Could you check a few things on this drawing? It's one solid part, dimensions in mm from its lowest x, y, z. A direction names the side the tool comes from. Give positions to 0.01 mm unless a question says otherwise; leave off trailing zeros. Loops run counter-clockwise (first coordinate to the right, second up) from the corner with the lowest first, then second, coordinate; pieces in that order, holes last.
Q1. Suppose I cut it at C-C (z = 7.5). List the corners of the cut face in (x, y) for me, and give its area (3 significant figures).
Q2. I need wall thicknesses on probe 1 along Z at (x, y) = (14, 30.5); probe 2 along Y at (x, z) = (14, 30) (1 decimal); probe 3 along Z at (x, y) = (36.5, 20). Which ranges of each line are inside material? Lowest first, please.
Q3. Suppose I cut it at D-D (x = 37). List the corners of the cut face in (y, z) for me.
Q4. I'm going to push flat-ended pins straight in: P1, Ø0.8, axis at x = 14.5, y = 5.5, coming from the +Z side; P2, Ø8, axis at x = 37, y = 13, coming from the +Z side; P3, Ø1.5, axis at x = 7.5, z = 22, coming from the +Y side. Where does each tip first touch, or does it pass through?
Q5. Suppose I cut it at A-A (x = 22). List the corners of the cut face in (y, z) for me, and give its area (3 significant figures).
Q6. Suppose I cut it at B-B (y = 19). List the corners of the cut face in (x, z) for me, and give its area (3 significant figures).
Q7. For the marked faces 1, 2 and 3, which set-ups out of +Z, -Z, +X, -X, +Y, -Y let a thin tool reach every point of the face, with its end or its side?
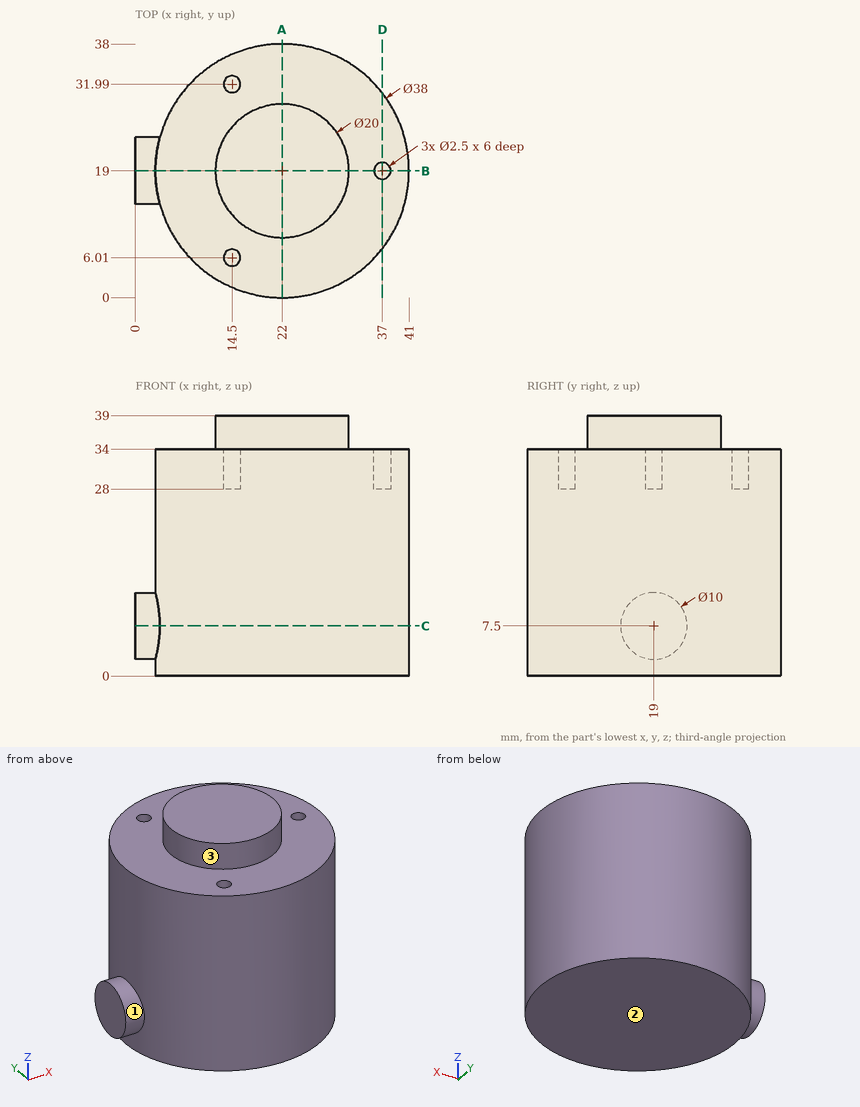
Solutions:
1. outline: (0, 14) - (3.67, 14) arc R19 ccw (long way) to (3.67, 24) - (0, 24) - close
1. area: 1,170 mm2
2. probe 1: z = 0 to 34
2. probe 2: y = 1.8 to 4.9, 7.2 to 30.8, 33.1 to 36.2
2. probe 3: z = 0 to 28
3. outline: (7.34, 0) - (30.66, 0) - (30.66, 34) - (20.25, 34) - (20.25, 28) - (17.75, 28) - (17.75, 34) - (7.34, 34) - close
4. P1: stops at z = 28
4. P2: stops at z = 34
4. P3: stops at y = 32.11
5. outline: (0, 0) - (38, 0) - (38, 34) - (29, 34) - (29, 39) - (9, 39) - (9, 34) - (0, 34) - close
5. area: 1,390 mm2
6. outline: (0, 2.5) - (3, 2.5) - (3, 0) - (41, 0) - (41, 34) - (38.25, 34) - (38.25, 28) - (35.75, 28) - (35.75, 34) - (32, 34) - (32, 39) - (12, 39) - (12, 34) - (3, 34) - (3, 12.5) - (0, 12.5) - close
6. area: 1,410 mm2
7. face 1: -X
7. face 2: -Z, +X, -X, +Y, -Y
7. face 3: +Z
